Design review of the part built by this model. Coordinates are the model's own, in mm. Face numbers are marked on the shaded views. A direction names the side the tool comes from. Coordinates: 2 decimals unless noted, no trailing zeros. Write each loop counter-clockwise with the first axis right and the second up, starting at its lowest first coordinate (ties: lowest second). Pieces come first, ordered by that corner, then holes.
Q1. For the marked faces 4, 5 and 6, list the 3-axis set-ups (+Z, -Z, +X, -X, +Y, -Y) from which the entire face can be reached by the end or side of a thin tool; tool diameter is ignored.
Q2. Take a section at D-D, the plane y = 21. Write out the cut boundary in (x, z), plus the area to 3 significant figures.
Q3. Take a section at C-C, the plane y = 1. Write out the cut boundary in (x, z).
Q4. For L1, parallel to X at y = 9.5, z = 19.5; L2, parallel to Y at x = -17, z = -2; L3, parallel to X at y = 13.75, z = 1, list the stretches that pass through material, from the lowest coordinate up.
Q5. Take a section at A-A, the plane x = 4.5. Write out the cut boundary in (y, z).
Q6. The part is to be moulded in two halves that separate along X. For the marked faces 1, 2 and 3, say which applies: released by +X, released by -X, zero draft, split by the parting line, or undercut.
Q7. For pin 1 Ø9 at (y, z) = (15, 16.5) entering from +X; pin 2 Ø3.5 at (y, z) = (11.5, 18) entering from -X; pin 3 Ø5 at (y, z) = (9.5, 6) entering from +X; pin 4 Ø5 at (x, z) = (-18, 4.5) entering from -Y, all flat-tipped, find the tip position at first contact; note any pin that passes through.
Q8. Take a section at B-B, the plane z = 17. Write out the cut boundary in (x, y), plus the area to 3 significant figures.
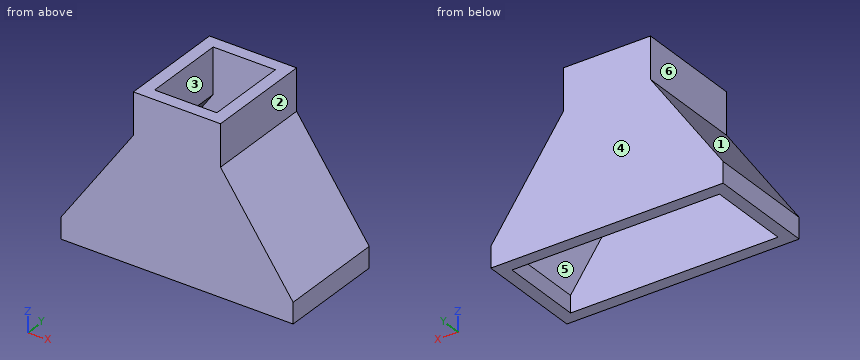
from build123d import *

# Parameters (mm, degrees)
SALIENTE_EXTRUIR1_DEPTH   = 20
SALIENTE_EXTRUIR1_2_DEPTH = 20
SALIENTE_EXTRUIR2_DEPTH   = 3
SALIENTE_EXTRUIR3_START   = -20
SALIENTE_EXTRUIR3_DEPTH   = 3


with BuildPart() as part:
    # Croquis1 → Saliente-Extruir1 (new body)
    with BuildSketch(Plane(origin=(0, 0, 0), x_dir=(1, 0, 0), z_dir=(0, 1, 0))):
        Polygon((-25, 17.391304348), (-25, 13.33697104), (-7.5, -11.66302896), (-7.5, -22.608695652), (-10.5, -22.608695652), (-10.5, -12.608695652), (-28, 12.391304348), (-28, 17.391304348), align=None)
    extrude(amount=SALIENTE_EXTRUIR1_DEPTH)



with BuildPart() as body_2:
    # Croquis1 → Saliente-Extruir1 2 (new body)
    with BuildSketch(Plane(origin=(0, 0, 0), x_dir=(1, 0, 0), z_dir=(0, 1, 0))):
        Polygon((7.5, -11.66302896), (7.5, -22.608695652), (10.5, -22.608695652), (10.5, -12.608695652), (28, 12.391304348), (28, 17.391304348), (25, 17.391304348), (25, 13.33697104), align=None)
    extrude(amount=SALIENTE_EXTRUIR1_2_DEPTH)


with BuildPart() as part_1:
    add(part.part)

    add(body_2.part)  # Saliente-Extruir2 merges body 2
    # Croquis2 → Saliente-Extruir2 (add)
    with BuildSketch(Plane(origin=(0, 20, 0), x_dir=(1, 0, 0), z_dir=(0, 1, 0))):
        Polygon((-10.5, -22.608695652), (10.5, -22.608695652), (10.5, -12.608695652), (28, 12.391304348), (28, 17.391304348), (-28, 17.391304348), (-28, 12.391304348), (-10.5, -12.608695652), align=None)
    extrude(amount=SALIENTE_EXTRUIR2_DEPTH)

    # Croquis2<2> → Saliente-Extruir3 (add)
    with BuildSketch(Plane(origin=(0, 20, 0), x_dir=(1, 0, 0), z_dir=(0, 1, 0)).offset(SALIENTE_EXTRUIR3_START)):
        Polygon((-10.5, -22.608695652), (10.5, -22.608695652), (10.5, -12.608695652), (28, 12.391304348), (28, 17.391304348), (-28, 17.391304348), (-28, 12.391304348), (-10.5, -12.608695652), align=None)
    extrude(amount=-SALIENTE_EXTRUIR3_DEPTH)


solid = part_1.part
Responses:
1. face 4: +Z, -Z, +X, -X, +Y
1. face 5: -Z
1. face 6: +Z, -X, +Y, -Y
2. outline: (-28, -17.39) - (28, -17.39) - (28, -12.39) - (10.5, 12.61) - (10.5, 22.61) - (-10.5, 22.61) - (-10.5, 12.61) - (-28, -12.39) - close
2. area: 1,450 mm2
3. outline: (-28, -17.39) - (-25, -17.39) - (-25, -13.34) - (-7.5, 11.66) - (-7.5, 22.61) - (-10.5, 22.61) - (-10.5, 12.61) - (-28, -12.39) - close; (7.5, 11.66) - (25, -13.34) - (25, -17.39) - (28, -17.39) - (28, -12.39) - (10.5, 12.61) - (10.5, 22.61) - (7.5, 22.61) - close
4. L1: x = -10.5 to -7.5, 7.5 to 10.5
4. L2: y = -3 to 0, 20 to 23
4. L3: x = -18.63 to -14.96, 14.96 to 18.63
5. outline: (-3, -17.39) - (0, -17.39) - (0, 22.61) - (-3, 22.61) - close; (20, -17.39) - (23, -17.39) - (23, 22.61) - (20, 22.61) - close
6. face 1: released by -X
6. face 2: released by +X
6. face 3: undercut
7. pin 1: stops at x = 10.93
7. pin 2: stops at x = -10.5
7. pin 3: stops at x = 16.88
7. pin 4: stops at y = -3
8. outline: (-10.5, -3) - (10.5, -3) - (10.5, 23) - (-10.5, 23) - close; hole (-7.5, 0) - (7.5, 0) - (7.5, 20) - (-7.5, 20) - close
8. area: 246 mm2
